Solid Edge part; units mm, degrees
sketch "Sketch1" plane through (0, 0, 0) normal (0, -1, 0) x (1, 0, 0)
  line L0 (-6, -20) -> (6, -20)
  line L1 (6, -20) -> (6, 20)
  line L2 (6, 20) -> (-6, 20)
  line L3 (-6, 20) -> (-6, -20)
  dimension "D1" = 6
  dimension "D2" = 6
extrude "Protrusion1" add sketch "Sketch1" against normal blind 5
fillet "Verrundung_3" radius 6 4 edges at (-6, 2.5, 20) (6, 2.5, 20) (-6, 2.5, -20) (6, 2.5, -20)
sketch "Sketch2" plane through (0, 5, 0) normal (0, 1, 0) x (0, 0, 1)
  circle A0 centre (-14, 0) radius 2.6
  circle A1 centre (14, 0) radius 2.6
extrude "Cutout1" cut sketch "Sketch2" against normal through all
chamfer "Chamfer1" distance 0.5 angle 45 3 edges at (0, 5, -16.6) (0, 0, 16.6) (0, 0, -11.4)
chamfer "Fase_7" distance 0.5 angle 45 1 edges at (0, 5, 11.4)
properties material "Nylon, allgemein"
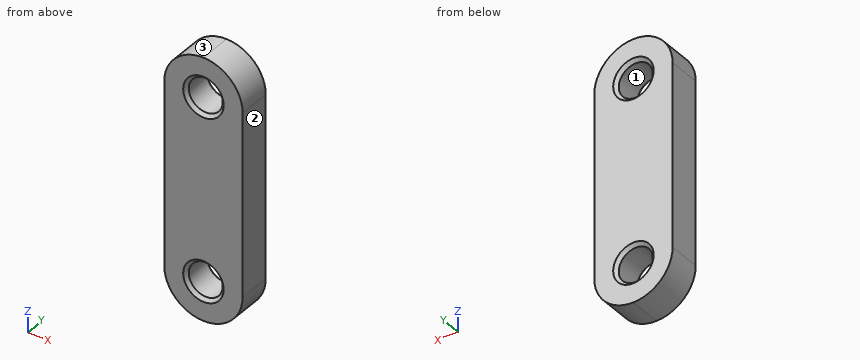
CAD build for the part. Positions are in the model's coordinates, mm. Face numbers are marked on the shaded views. Round coordinates to 2 decimals unless told otherwise and drop trailing zeros. Write each loop counter-clockwise with the first axis right and the second up, starting at its lowest first coordinate (ties: lowest second). Pieces come first, ordered by that corner, then holes. Notation, with made-up numbers: M 75.25,-29 L 91.25,-29 A18 ccw 91.25,1 Z; hole C -10.5,-2 d6. An arc over 180 degrees is marked long. Use a Markdown table: item, result. Add a question column.
1. Flat gauge pins, fed straight in: P1, Ø2, axis at x = 3.5, y = 4, coming from the -Z side; P2, Ø2, axis at x = 4.5, y = 1, coming from the -Z side. Where does each tip first touch, or does it go through?
2. Slice it at B-B on x = 5. Give the cut face in (y, z), then the cut area to 3 significant figures.
3. Pull direction Z, two halves, no side cores. Call the marked faces 1, 2 and 3: released by +Z, released by -Z, zero draft, split by the parting line, or undercut.
4. Slice it at C-C on x = -4.5. Give the cut face in (y, z).
5. Slice it at A-A on y = 2.05. Give the number of separate pieces and of enclosed holes in the cut face, then the cut area to 3 significant figures.
6. Drill centre lines: probe 1 along X at (y, z) = (3.3, -14); probe 2 along Z at (x, y) = (-1, 2.85); probe 3 along Z at (x, y) = (2, 1.55). Where is each one in solid material? Low to high.
Reply:
| question | item | result |
|---|---|---|
| 1 | P1 | stops at z = -19.45 |
| 1 | P2 | stops at z = -18.87 |
| 2 | outline | M 0,-17.32 L 5,-17.32 L 5,17.32 L 0,17.32 Z |
| 2 | area | 173 mm^2 |
| 3 | face 1 | undercut |
| 3 | face 2 | zero draft |
| 3 | face 3 | released by +Z |
| 4 | outline | M 0,-17.97 L 5,-17.97 L 5,17.97 L 0,17.97 Z |
| 5 | separate pieces | 1 |
| 5 | enclosed holes | 2 |
| 5 | area | 407 mm^2 |
| 6 | probe 1 | x = -6 to -2.6, 2.6 to 6 |
| 6 | probe 2 | z = -19.92 to -16.4, -11.6 to 11.6, 16.4 to 19.92 |
| 6 | probe 3 | z = -19.66 to -15.66, -12.34 to 12.34, 15.66 to 19.66 |
